from build123d import *

# Parameters (mm, degrees)
F0_R     = 6
F1_DEPTH = 6
F3_DEPTH = 4
F4_R     = 5
F5_DEPTH = 16
F6_R     = 2.5
F7_DEPTH = 22.001
F8_SIZE  = 0.5


with BuildPart() as f1:
    # F0 (on Front) → F1 (new body)
    with BuildSketch(Plane.XZ):
        Circle(F0_R)
    extrude(amount=-F1_DEPTH)

    # F2 (on face) → F3 (cut)
    with BuildSketch(Plane.XZ):
        Polygon((3.708328, 2.753478), (-0.530418, 4.588245), (-4.238745, 1.834767), (-3.708328, -2.753478), (0.530418, -4.588245), (4.238745, -1.834767), align=None)
    extrude(amount=-F3_DEPTH, mode=Mode.SUBTRACT)

    # F4 (on face) → F5 (join)
    with BuildSketch(Plane(origin=(0, 6, 0), x_dir=(-1, 0, 0), z_dir=(0, 1, 0))):
        Circle(F4_R)
    extrude(amount=F5_DEPTH)

    # F6 (on face) → F7 (cut, through all)
    with BuildSketch(Plane(origin=(0, 22, 0), x_dir=(-1, 0, 0), z_dir=(0, 1, 0))):
        Circle(F6_R)
    extrude(amount=-F7_DEPTH, mode=Mode.SUBTRACT)

    # F8
    f8_edges = [f1.edges().sort_by_distance(p)[0] for p in [
        (-6, 0, 0),
        (6, 3, 0),
        (-6, 6, 0),
        (5, 22, 0),
    ]]
    chamfer(f8_edges, length=F8_SIZE)


solid = f1.part
Source: CAD feature listing. Evaluate the final solid. Frame: model axes, mm. A direction names the side the tool comes from. Round coordinates to 2 decimals unless told otherwise and drop trailing zeros. Write each loop counter-clockwise with the first axis right and the second up, starting at its lowest first coordinate (ties: lowest second). Pieces come first, ordered by that corner, then holes. Notation, with made-up numbers: (50.25, 37.5) - (61.25, 37.5) arc R22 cw to (61.25, 70.5) - close; hole circle Ø3 at (53.25, -12.5). An arc over 180 degrees is marked (long way). Use CSV: the item, a comma, the result in double quotes. Start each with the question number.
(1) First-contact query: pin 1 Ø6 at (x, z) = (0, 0) entering from -Y; pin 2 Ø6 at (x, z) = (4.5, -0.5) entering from +Y; pin 3 Ø4 at (x, y) = (-5, 18.5) entering from +Z; pin 4 Ø3 at (y, z) = (10, -1.5) entering from -X. Flat tips, straight axial feed; report the tip coordinate or a pass-through.
(2) Cut plane C-C, the plane z = 0. Return loops of the section in (x, y).
(3) Material intervals for probe 1 along Z at (x, y) = (0, 15.75); probe 2 along Y at (x, z) = (-4.5, -3); probe 3 along Y at (x, z) = (-3.5, -0.75), sorted ascending. Write a range as [from, to].
(4) Cut plane A-A, the plane y = 3.75. Return loops of the section in (x, z).
(5) Mould query, pull axis X, two halves, no side actions, for faces 1 (the face through (1.619, 1.972, 3.658)), 2 (the face through (1.08, 13.64, -4.88)), 3 (the face through (2, 0, 4)). Classes: pulls with the +X half, pulls with the -X half, needs draft (parallel to the pull), parting line crosses it, or undercut.
(6) Cut plane B-B, the plane x = 0. Return loops of the section in (y, z), and give its area (3 significant figures).
(7) Cut plane D-D, the plane y = 14.75. Return loops of the section in (x, z).
(8) Set-up query: faces 4 (the face through (-6, 3, 0)), 5 (the face through (-2.4, 2, 3.2)), 6 (the face through (1.6, 6, -4.9)). Return all of +Z, -Z, +X, -X, +Y, -Y with unobstructed straight access to the full face (end or side cutting, diameter ignored); none if empty.
Geometry says:
1,pin 1,"y = 4"
1,pin 2,"y = 22"
1,pin 3,"z = 4"
1,pin 4,"x = -5"
2,outline,"(-6, 0.5) - (-5.5, 0) - (-4.03, 0) - (-4.03, 4) - (-2.5, 4) - (-2.5, 22) - (-4.5, 22) - (-5, 21.5) - (-5, 6) - (-5.5, 6) - (-6, 5.5) - close; (2.5, 4) - (4.03, 4) - (4.03, 0) - (5.5, 0) - (6, 0.5) - (6, 5.5) - (5.5, 6) - (5, 6) - (5, 21.5) - (4.5, 22) - (2.5, 22) - close"
3,probe 1,"[-5, -2.5], [2.5, 5]"
3,probe 2,"[0, 6]"
3,probe 3,"[4, 22]"
4,outline,"circle Ø12 at (0, 0); hole (-4.24, 1.83) - (-3.71, -2.75) - (0.53, -4.59) - (4.24, -1.83) - (3.71, 2.75) - (-0.53, 4.59) - close"
5,face 1,"undercut"
5,face 2,"parting line crosses it"
5,face 3,"needs draft"
6,outline,"(0, -5.5) - (0.5, -6) - (5.5, -6) - (6, -5.5) - (6, -5) - (21.5, -5) - (22, -4.5) - (22, -2.5) - (4, -2.5) - (4, -4.36) - (0, -4.36) - close; (0, 4.36) - (4, 4.36) - (4, 2.5) - (22, 2.5) - (22, 4.5) - (21.5, 5) - (6, 5) - (6, 5.5) - (5.5, 6) - (0.5, 6) - (0, 5.5) - close"
6,area,"106 mm²"
7,outline,"circle Ø10 at (0, 0); hole circle Ø5 at (0, 0)"
8,face 4,"+Y, -Y"
8,face 5,"-Y"
8,face 6,"+Y"
